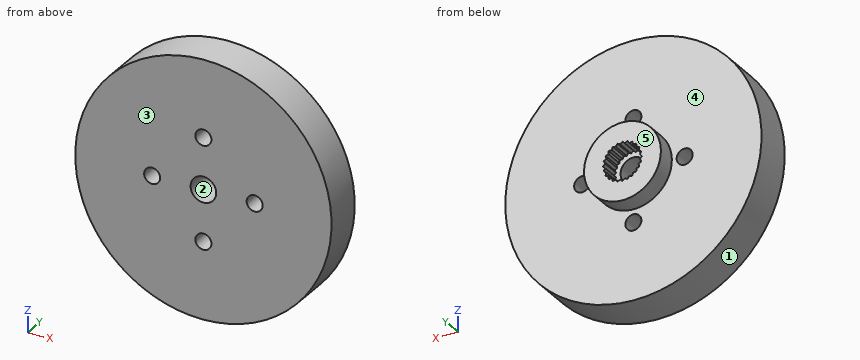
```python
from build123d import *

# Parameters (mm, degrees)
SKETCH1_R           = 6
BOSS_EXTRUDE1_DEPTH = 3
SKETCH2_R           = 20
SKETCH2_R_2         = 2
SKETCH2_R_3         = 1.25
BOSS_EXTRUDE2_DEPTH = 6.35


with BuildPart() as part:
    # Sketch1 → Boss-Extrude1 (new body)
    with BuildSketch(Plane(origin=(0, 0, 0), x_dir=(1, 0, 0), z_dir=(0, 1, 0))):
        with Locations(Location((-0.004099667, 0.000679594, 0), (0, 0, 270))):
            Circle(SKETCH1_R)
        Polygon((-0.004099667, 3.041629594), (-0.360179239, 2.705372466), (-0.791155443, 2.938011735), (-1.048072148, 2.521052117), (-1.524574667, 2.634219546), (-1.664820058, 2.164972545), (-2.154376034, 2.15095596), (-2.168392618, 1.661399985), (-2.637639619, 1.521154594), (-2.52447219, 1.044652075), (-2.941431809, 0.787735369), (-2.708792539, 0.356759166), (-3.045049667, 0.000679594), (-2.708792539, -0.355399978), (-2.941431809, -0.786376181), (-2.52447219, -1.043292887), (-2.637639619, -1.519795406), (-2.168392618, -1.660040797), (-2.154376034, -2.149596772), (-1.664820058, -2.163613357), (-1.524574667, -2.632860358), (-1.048072148, -2.519692929), (-0.791155443, -2.936652547), (-0.360179239, -2.704013278), (-0.004099667, -3.040270406), (0.351979904, -2.704013278), (0.782956108, -2.936652547), (1.039872814, -2.519692929), (1.516375333, -2.632860358), (1.656620724, -2.163613357), (2.146176699, -2.149596772), (2.160193283, -1.660040797), (2.629440284, -1.519795406), (2.516272855, -1.043292887), (2.933232474, -0.786376181), (2.700593205, -0.355399978), (3.036850333, 0.000679594), (2.700593205, 0.356759166), (2.933232474, 0.787735369), (2.516272855, 1.044652075), (2.629440284, 1.521154594), (2.160193283, 1.661399985), (2.146176699, 2.15095596), (1.656620724, 2.164972545), (1.516375333, 2.634219546), (1.039872814, 2.521052117), (0.782956108, 2.938011735), (0.351979904, 2.705372466), align=None, mode=Mode.SUBTRACT)
    extrude(amount=BOSS_EXTRUDE1_DEPTH)

    # Sketch2 → Boss-Extrude2 (add)
    with BuildSketch(Plane.XZ):
        with Locations(Location((0, 0, 0), (0, 0, 270))):
            Circle(SKETCH2_R)
        with Locations(Location((0, 0, 0), (0, 0, 270))):
            Circle(SKETCH2_R_2, mode=Mode.SUBTRACT)
        with Locations(Location((8, 0, 0), (0, 0, 270))):
            Circle(SKETCH2_R_3, mode=Mode.SUBTRACT)
        with Locations(Location((0, -8, 0), (0, 0, 270))):
            Circle(SKETCH2_R_3, mode=Mode.SUBTRACT)
        with Locations(Location((-8, 0, 0), (0, 0, 270))):
            Circle(SKETCH2_R_3, mode=Mode.SUBTRACT)
        with Locations(Location((0, 8, 0), (0, 0, 270))):
            Circle(SKETCH2_R_3, mode=Mode.SUBTRACT)
    extrude(amount=BOSS_EXTRUDE2_DEPTH)


solid = part.part
```
Build history of the part. All positions in model axes, mm. Face numbers are marked on the shaded views. A direction names the side the tool comes from. Give positions to 0.01 mm unless a question says otherwise; leave off trailing zeros. Loops run counter-clockwise (first coordinate to the right, second up) from the corner with the lowest first, then second, coordinate; pieces in that order, holes last.
1) Drop flat-ended pins along their axis: P1, Ø3, axis at x = -5.5, y = 0.5, coming from the +Z side; P2, Ø2, axis at x = -8, y = -1.5, coming from the -Z side (3 decimals); P3, Ø5, axis at x = 6, z = -11.5, coming from the +Y side; P4, Ø6.5, axis at x = 1, z = -0.5, coming from the +Y side. Give the stop position or say it passes through.
Values follow:
P1: stops at z = 19.58
P2: stops at z = -18.735
P3: stops at y = 0
P4: stops at y = 3
2) Two-plate mould, pull along Z, no slides. Class the marked faces 1, 2 and 3: released by +Z, released by -Z, zero draft, split by the parting line, or undercut.
Values follow:
face 1: split by the parting line
face 2: undercut
face 3: zero draft
3) Band-saw the part on D-D on z = 14. List the corners of the cut face in (x, y).
Values follow:
outline: (-14.28, -6.35) - (14.28, -6.35) - (14.28, 0) - (-14.28, 0) - close
4) Band-saw the part on B-B on y = -1.25. List the corners of the cut face in (x, z).
Values follow:
outline: circle Ø40 at (0, 0); hole circle Ø2.5 at (-8, 0); hole circle Ø4 at (0, 0); hole circle Ø2.5 at (0, -8); hole circle Ø2.5 at (0, 8); hole circle Ø2.5 at (8, 0)
5) Band-saw the part on C-C on x = 8. List the corners of the cut face in (y, z), then the cut area to 3 significant figures.
Values follow:
outline: (-6.35, -18.33) - (0, -18.33) - (0, -1.25) - (-6.35, -1.25) - close; (-6.35, 1.25) - (0, 1.25) - (0, 18.33) - (-6.35, 18.33) - close
area: 217 mm2
6) 3-axis set-ups, long thin cutter, end or side, ignore diameter. For the marked faces 4 and 5: which of +Z, -Z, +X, -X, +Y, -Y reach the whole face in a straight line?
Values follow:
face 4: +Y
face 5: +Z, -Z, +X, -X, +Y
7) Band-saw the part on A-A on z = 8. List the corners of the cut face in (x, y).
Values follow:
outline: (-18.33, -6.35) - (-1.25, -6.35) - (-1.25, 0) - (-18.33, 0) - close; (1.25, -6.35) - (18.33, -6.35) - (18.33, 0) - (1.25, 0) - close
8) Probe line 1 along Y through (x, z) = (-13.5, -6); line 2 along X through (y, z) = (-2, -8); line 3 along X through (y, z) = (2, -0.5). List the from-to ranges inside material, lowest first.
Values follow:
line 1: y = -6.35 to 0
line 2: x = -18.33 to -1.25, 1.25 to 18.33
line 3: x = -5.98 to -2.79, 2.78 to 5.98
